```python
from build123d import *


with BuildPart() as f1:
    # F0 (on Front) → F1 (revolve)
    with BuildSketch(Plane.XZ):
        with BuildLine():
            Line((0, 76.2), (0, 0))
            Line((0, 0), (6.35, 0))
            ThreePointArc((6.35, 0), (8.5950640303, 0.9299359697), (9.525, 3.175))
            Line((9.525, 3.175), (9.525, 6.35))
            Line((9.525, 6.35), (3.175, 6.35))
            Line((3.175, 6.35), (3.175, 8.35))
            Line((3.175, 8.35), (9.525, 8.35))
            Line((9.525, 8.35), (9.525, 14.7))
            add(Edge.make_bspline(
                [(0, 76.2), (3.168798384, 76.1437072296), (11.1827318992, 76.0013439789), (11.5605251086, 51.7730056699), (2.8817099393, 39.4723955532), (11.6856190133, 21.9527870322), (10.1300446041, 16.7310482843), (9.525, 14.7)],
                knots=[0, 0, 0, 0, 0.1621620078, 0.4101099439, 0.6253550155, 0.854278438, 1, 1, 1, 1], degree=3))
        make_face()
    revolve(axis=Axis((0, 0, 38.1), (0, 0, 1)))


solid = f1.part
```
Geometry check sheet. Reference: the model listing, model coordinates, mm. A direction names the side the tool comes from. Coordinates: 2 decimals unless noted, no trailing zeros. Answer in a Markdown table with one row per item. Add a question column.
1. Section check A-A (x = -7.75). Give the number of separate pieces and of enclosed holes in the cut face, plus the area to 3 significant figures.
2. Access from +Z, -Z, +X, -X, +Y, -Y to the whole of each face (thin tool, end or side, straight path). Record for faces 1 (the face through (-4, 0, 8.35)), 2 (the face through (0, 0, 0)), 3 (the face through (-7.559, -5.796, 11.569)).
3. Gauge pin test, flat ends, axial feed: pin 1 Ø2 at (x, z) = (3, 52.5) entering from +Y; pin 2 Ø6 at (y, z) = (7.5, 31.5) entering from -X; pin 3 Ø1 at (y, z) = (-4, 43.5) entering from -X. Record the tip position at first contact, or that the pin passes through.
4. Material ranges on L1, parallel to Z at x = -3.5, y = 3.5; L2, parallel to Z at x = -4.5, y = 3; L3, parallel to X at y = 6.5, z = 56, recorded low to high. Write a range as [from, to].
Data:
| question | item | result |
|---|---|---|
| 1 | separate pieces | 3 |
| 1 | enclosed holes | 0 |
| 1 | area | 630 mm² |
| 2 | face 1 | none |
| 2 | face 2 | -Z, +X, -X, +Y, -Y |
| 2 | face 3 | -Z |
| 3 | pin 1 | stops at y = 9.54 |
| 3 | pin 2 | stops at x = -6.07 |
| 3 | pin 3 | stops at x = -5.67 |
| 4 | L1 | z = [0, 6.35], [8.35, 75.72] |
| 4 | L2 | z = [0, 6.35], [8.35, 75.58] |
| 4 | L3 | x = [-8.06, 8.06] |
